CAD build for the part. Positions are in the model's coordinates, mm. Coordinates: 2 decimals unless noted, no trailing zeros. Write each loop counter-clockwise with the first axis right and the second up, starting at its lowest first coordinate (ties: lowest second). Pieces come first, ordered by that corner, then holes. Notation, with made-up numbers: (55, 40) - (102, 40) arc R26 ccw to (102, 61) - close; hole circle Ø6 at (53, 54). An arc over 180 degrees is marked (long way). Answer in a Markdown table with one row per item. Add a question column.
Q1. Band-saw the part on A-A (x = 400). List the corners of the cut face in (y, z), and give its area (3 significant figures).
Q2. Two-plate mould, pull along Y, no slides. Class faces 1 (the flat face through (104, 0, -4.5)), 2 (the cylindrical face through (-193.534, -2.681, -0.063)), 3 (the cylindrical face through (406.677, 2.103, -0.063)): +Y half, -Y half, draft (parallel to the pull), parting line (faces both ways), or undercut.
Q3. Drill centre lines: line 1 along Y through (x, z) = (0, -0.25); line 2 along X through (y, z) = (-1, -3.75); line 3 along X through (y, z) = (-4.25, -1.75). Where is each one in solid material? Low to high. Write a range as from..to.
Q4. Pin check, flat tip, straight feed: pin 1 (4 mm diameter, centred on y = -8.5, z = 0, fed in from +X). Stop position of the tip, or through.
Q5. Band-saw the part on B-B (z = 1). List the corners of the cut face in (x, y), and give its area (3 significant figures).
```python
from build123d import *

# Parameters (mm, degrees)
SKETCH_1_R      = 7
EXTRUDE_1_DEPTH = 4.5


with BuildPart() as part:
    # 草圖1 → 填料-伸長1 (new body, symmetric)
    with BuildSketch(Plane.XY):
        Polygon((-215, 7.5), (-210, 12.5), (410, 12.5), (415, 7.5), (415, -7.5), (410, -12.5), (-210, -12.5), (-215, -7.5), align=None)
        Circle(SKETCH_1_R, mode=Mode.SUBTRACT)
        with Locations((400, 0)):
            Circle(SKETCH_1_R, mode=Mode.SUBTRACT)
        with Locations((-200, 0)):
            Circle(SKETCH_1_R, mode=Mode.SUBTRACT)
    extrude(amount=EXTRUDE_1_DEPTH, both=True)


solid = part.part
```
Checked values:
| question | item | result |
|---|---|---|
| 1 | outline | (-12.5, -4.5) - (-7, -4.5) - (-7, 4.5) - (-12.5, 4.5) - close; (7, -4.5) - (12.5, -4.5) - (12.5, 4.5) - (7, 4.5) - close |
| 1 | area | 99.0 mm² |
| 2 | face 1 | draft |
| 2 | face 2 | undercut |
| 2 | face 3 | undercut |
| 3 | line 1 | y = -12.5..-7, 7..12.5 |
| 3 | line 2 | x = -215..-206.93, -193.07..-6.93, 6.93..393.07, 406.93..415 |
| 3 | line 3 | x = -215..-205.56, -194.44..-5.56, 5.56..394.44, 405.56..415 |
| 4 | pin 1 | stops at x = 415 |
| 5 | outline | (-215, -7.5) - (-210, -12.5) - (410, -12.5) - (415, -7.5) - (415, 7.5) - (410, 12.5) - (-210, 12.5) - (-215, 7.5) - close; hole circle Ø14 at (-200, 0); hole circle Ø14 at (0, 0); hole circle Ø14 at (400, 0) |
| 5 | area | 15,200 mm² |
